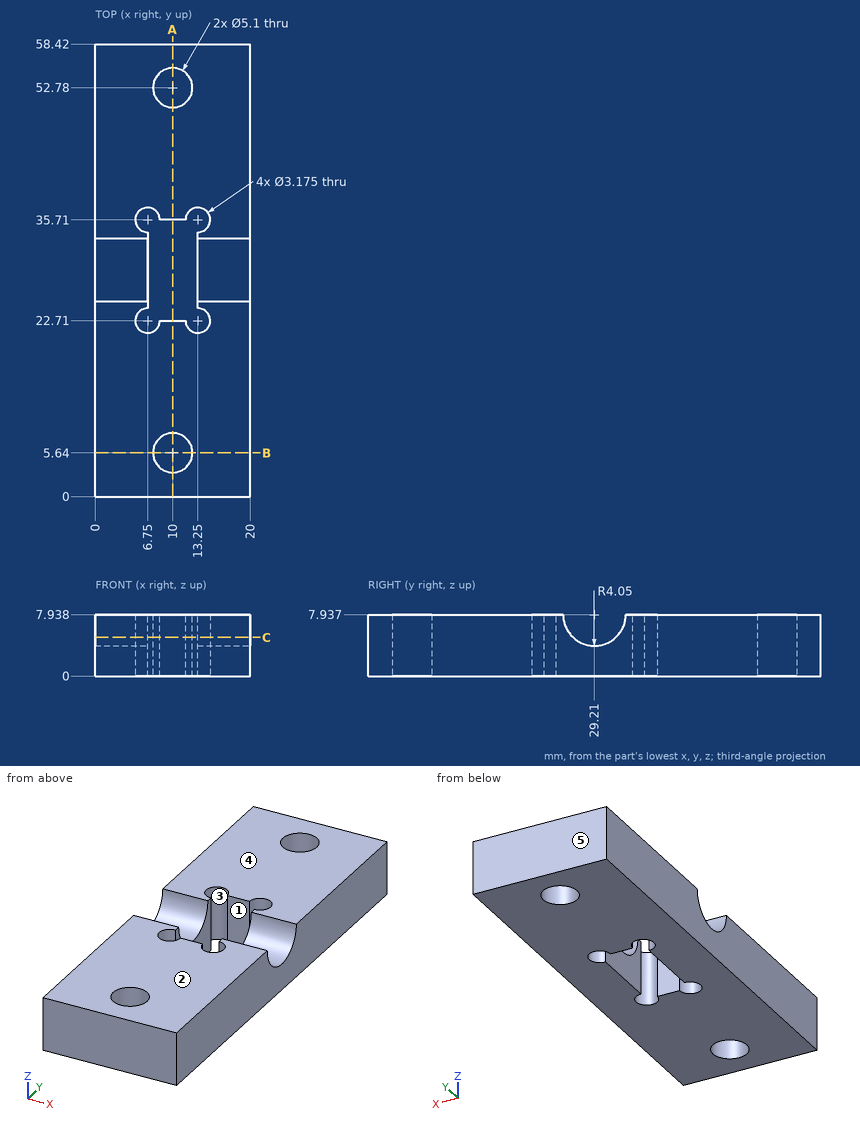
Geometry check sheet. Reference: drawing and pictorial views, mm from the part's lowest x, y, z. A direction names the side the tool comes from. Round coordinates to 2 decimals unless told otherwise and drop trailing zeros. Loops run counter-clockwise (first coordinate to the right, second up) from the corner with the lowest first, then second, coordinate; pieces in that order, holes last. Notation, with made-up numbers: (49, 18) - (108, 18) arc R22 ccw to (108, 49) - close; hole circle Ø4 at (13, 63). An arc over 180 degrees is marked (long way). Write item = value, one per line. Start each with the question number.
Q1. Section check C-C (z = 5). Count the separate pieces of the cut face and the enclosed holes in it, plus the area to 3 significant figures.
Q2. Access from +Z, -Z, +X, -X, +Y, -Y to the whole of each face (thin tool, end or side, straight path). Record for the marked faces 1 and 2.
Q3. Section check B-B (y = 5.64). Record the boundary of the cut face in (x, z), plus the area to 3 significant figures.
Q4. Section check A-A (x = 10). Record the boundary of the cut face in (y, z).
Q5. Thickness scan on L1, parallel to Y at x = 9.75, z = 5.25; L2, parallel to X at y = 29.5, z = 3.5; L3, parallel to Y at x = 12, z = 1 (1 decimal). Record the ranges inside material, lowest first.
Q6. Release check for a two-part mould opening along Y. For the marked faces 3, 4 and 5 record: pulls with the +Y half, pulls with the -Y half, needs draft (parallel to the pull), parting line crosses it, or undercut.
Derived:
q1.separate_pieces = 2
q1.enclosed_holes = 2
q1.area = 944 mm^2
q2.face_1 = +Z, -Z
q2.face_2 = +Z, +X, -X, +Y, -Y
q3.outline = (0, 0) - (7.45, 0) - (7.45, 7.94) - (0, 7.94) - close; (12.55, 0) - (20, 0) - (20, 7.94) - (12.55, 7.94) - close
q3.area = 118 mm^2
q4.outline = (0, 0) - (3.09, 0) - (3.09, 7.94) - (0, 7.94) - close; (8.19, 0) - (22.71, 0) - (22.71, 7.94) - (8.19, 7.94) - close; (35.71, 0) - (50.23, 0) - (50.23, 7.94) - (35.71, 7.94) - close; (55.33, 0) - (58.42, 0) - (58.42, 7.94) - (55.33, 7.94) - close
q5.L1 = 0 to 3.1, 8.18 to 22.71, 35.71 to 50.24, 55.32 to 58.42
q5.L2 = 0 to 6.75, 13.25 to 20
q5.L3 = 0 to 4.1, 7.2 to 21.7, 36.7 to 51.2, 54.4 to 58.4
q6.face_3 = undercut
q6.face_4 = needs draft
q6.face_5 = pulls with the +Y half
